```python
from build123d import *

# Parameters (mm, degrees)
ESBO_O1_R                  = 15
RESSALTO_EXTRUS_O1_DEPTH   = 30
ESBO_O2_R                  = 10
CORTE_EXTRUS_O1_DEPTH      = 15
RESSALTO_EXTRUS_O2_DEPTH   = 10
ESBO_O4_R                  = 1
CORTE_EXTRUS_O2_DEPTH      = 5
ESBO_O5_R                  = 3.5
CORTE_EXTRUS_O3_DEPTH      = 20
ESBO_O6_R                  = 2
CORTE_EXTRUS_O4_DEPTH      = 16
CORTE_EXTRUS_O4_DEPTH_BACK = 16
ESBO_O7_R                  = 2.5
CORTE_EXTRUS_O5_DEPTH      = 16.0000001
CORTE_EXTRUS_O6_DEPTH      = 4
FILETE1_R                  = 1
FILETE2_R                  = 3
FILETE4_R                  = 1


with BuildPart() as part:
    # Esboço1 → Ressalto-extrusão1 (new body)
    with BuildSketch(Plane(origin=(0, 0, 0), x_dir=(1, 0, 0), z_dir=(0, 1, 0))):
        Circle(ESBO_O1_R)
    extrude(amount=RESSALTO_EXTRUS_O1_DEPTH)

    # Esboço2 → Corte-extrusão1 (cut)
    with BuildSketch(Plane(origin=(0, 30, 0), x_dir=(1, 0, 0), z_dir=(0, 1, 0))):
        Circle(ESBO_O2_R)
    extrude(amount=-CORTE_EXTRUS_O1_DEPTH, mode=Mode.SUBTRACT)

    # Esboço3 → Ressalto-extrusão2 (add)
    with BuildSketch(Plane.XZ):
        with BuildLine():
            Line((-5, -8.660254038), (5, -8.660254038))
            ThreePointArc((5, -8.660254038), (10, 0), (5, 8.660254038))
            Line((5, 8.660254038), (-5, 8.660254038))
            ThreePointArc((-5, 8.660254038), (-10, 0), (-5, -8.660254038))
        make_face()
    extrude(amount=RESSALTO_EXTRUS_O2_DEPTH)

    # Esboço4 → Corte-extrusão2 (cut)
    with BuildSketch(Plane.XZ.offset(10)):
        Circle(ESBO_O4_R)
    extrude(amount=-CORTE_EXTRUS_O2_DEPTH, mode=Mode.SUBTRACT)

    # Esboço5 → Corte-extrusão3 (cut)
    with BuildSketch(Plane(origin=(0, 15, 0), x_dir=(1, 0, 0), z_dir=(0, 1, 0))):
        Circle(ESBO_O5_R)
    extrude(amount=-CORTE_EXTRUS_O3_DEPTH, mode=Mode.SUBTRACT)

    # Esboço6 → Corte-extrusão4 (cut, two sides)
    with BuildSketch(Plane.XY) as corte_extrus_o4_sk:
        with Locations((0, 22.5)):
            Circle(ESBO_O6_R)
    extrude(amount=CORTE_EXTRUS_O4_DEPTH, mode=Mode.SUBTRACT)
    extrude(corte_extrus_o4_sk.sketch, amount=-CORTE_EXTRUS_O4_DEPTH_BACK, mode=Mode.SUBTRACT)

    # Esboço7 → Corte-extrusão5 (cut, through all)
    with BuildSketch(Plane(origin=(0, 0, 0), x_dir=(0, 0, -1), z_dir=(1, 0, 0))):
        with Locations((0, 17.5)):
            Circle(ESBO_O7_R)
    extrude(amount=-CORTE_EXTRUS_O5_DEPTH, mode=Mode.SUBTRACT)

    # Esboço9 → Corte-extrusão6 (cut)
    with BuildSketch(Plane.XZ.offset(10)):
        with BuildLine():
            Line((2.645751311, 3), (2.645751311, -3))
            ThreePointArc((2.645751311, -3), (-4, 0), (2.645751311, 3))
        make_face()
    extrude(amount=-CORTE_EXTRUS_O6_DEPTH, mode=Mode.SUBTRACT)

    # Filete1
    filete1_edges = [part.edges().sort_by_distance(p)[0] for p in [
        (-15, 30, 0),
    ]]
    fillet(filete1_edges, radius=FILETE1_R)

    # Filete2
    filete2_edges = [part.edges().sort_by_distance(p)[0] for p in [
        (-15, 0, 0),
    ]]
    fillet(filete2_edges, radius=FILETE2_R)

    # Filete4
    filete4_edges = [part.edges().sort_by_distance(p)[0] for p in [
        (-5, -5, 8.660254038),
        (-5, -5, -8.660254038),
        (5, -5, -8.660254038),
        (5, -5, 8.660254038),
    ]]
    fillet(filete4_edges, radius=FILETE4_R)


solid = part.part
```
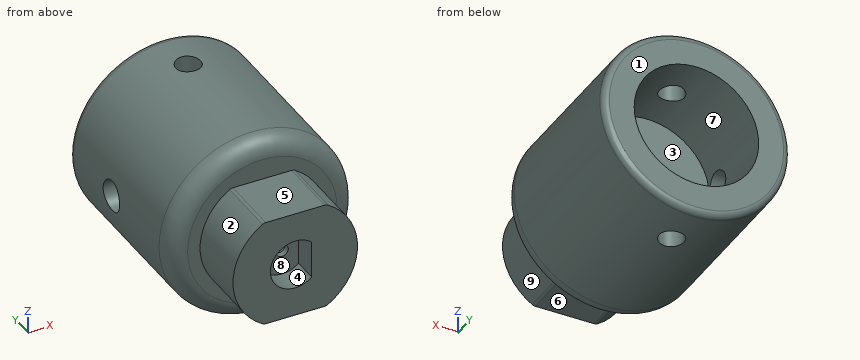
Check sheet for the modelled part. Datum: model origin and axes. Units: mm. Face numbers are marked on the shaded views. A direction names the side the tool comes from. Coordinates: 2 decimals unless noted, no trailing zeros. Loops run counter-clockwise (first coordinate to the right, second up) from the corner with the lowest first, then second, coordinate; pieces in that order, holes last. Notation, with made-up numbers: M 33,-18.5 L 82,-18.5 A6 ccw 82,-8.5 Z; hole C 61.25,-13.75 d11. An arc over 180 degrees is marked long. Answer as a JSON object with one key per item and string values.
1. Sectioned sample at C-C on x = 0. Count the separate pieces of the cut face and the enclosed holes in it, and give its area (3 significant figures).
Outcome:
{"separate pieces": "4", "enclosed holes": "0", "area": "555 mm²"}
2. Scan lines: L1, parallel to Z at x = 0, y = -5.6; L2, parallel to Y at x = 0, z = 12.25; L3, parallel to X at y = 24.25, z = 0. Record each from-to range of solid material in increasing order. Write a range as from..to.
Outcome:
{"L1": "-8.66..-1, 1..8.66", "L2": "0.01..20.5, 24.5..30", "L3": "-15..-10, 10..15"}
3. Sectioned sample at A-A on y = -5.5. Record the cut outline in (x, z).
Outcome:
{"outline": "M -5.25,-8.51 A1 ccw -4.72,-8.66 L 4.72,-8.66 A1 ccw 5.25,-8.51 A10 ccw 5.25,8.51 A1 ccw 4.72,8.66 L -4.72,8.66 A1 ccw -5.25,8.51 A10 ccw Z; hole C 0,0 d2"}
4. Sectioned sample at D-D on y = 17.5. Record the cut outline in (x, z).
Outcome:
{"outline": "M -14.79,-2.5 A15 ccw long -14.79,2.5 L -9.68,2.5 A10 cw long -9.68,-2.5 Z"}
5. Access from +Z, -Z, +X, -X, +Y, -Y to the whole of each face (thin tool, end or side, straight path). Record for the marked faces 5, 6, 7, 8 and 9.
Outcome:
{"face 5": "+Z, +X, -X, -Y", "face 6": "-Z, +X, -X, -Y", "face 7": "+Y", "face 8": "-Y", "face 9": "+X, -Y"}
6. Sectioned sample at B-B on y = 22.5. Record the cut outline in (x, z).
Outcome:
{"outline": "M -2,-14.87 L -2,-9.8 A10 cw -2,9.8 L -2,14.87 A15 ccw Z; M 2,-14.87 A15 ccw 2,14.87 L 2,9.8 A10 cw 2,-9.8 Z"}
7. Release check for a two-part mould opening along X. For the marked faces 1, 2, 3 and 4 record: pulls with the +X half, pulls with the -X half, needs draft (parallel to the pull), parting line crosses it, or undercut.
Outcome:
{"face 1": "needs draft", "face 2": "pulls with the -X half", "face 3": "undercut", "face 4": "undercut"}
8. Depth check by flat-ended pin: P1, Ø6, axis at x = -1.5, z = -1, coming from the +Y side; P2, Ø4.5, axis at x = 1.5, y = -3.5, coming from the -Z side; P3, Ø6, axis at x = -7.5, y = 14, coming from the -Z side. Enter the tip coordinate at first touch or a pass-through.
Outcome:
{"P1": "y = 15", "P2": "z = -8.66", "P3": "z = -14.31"}
